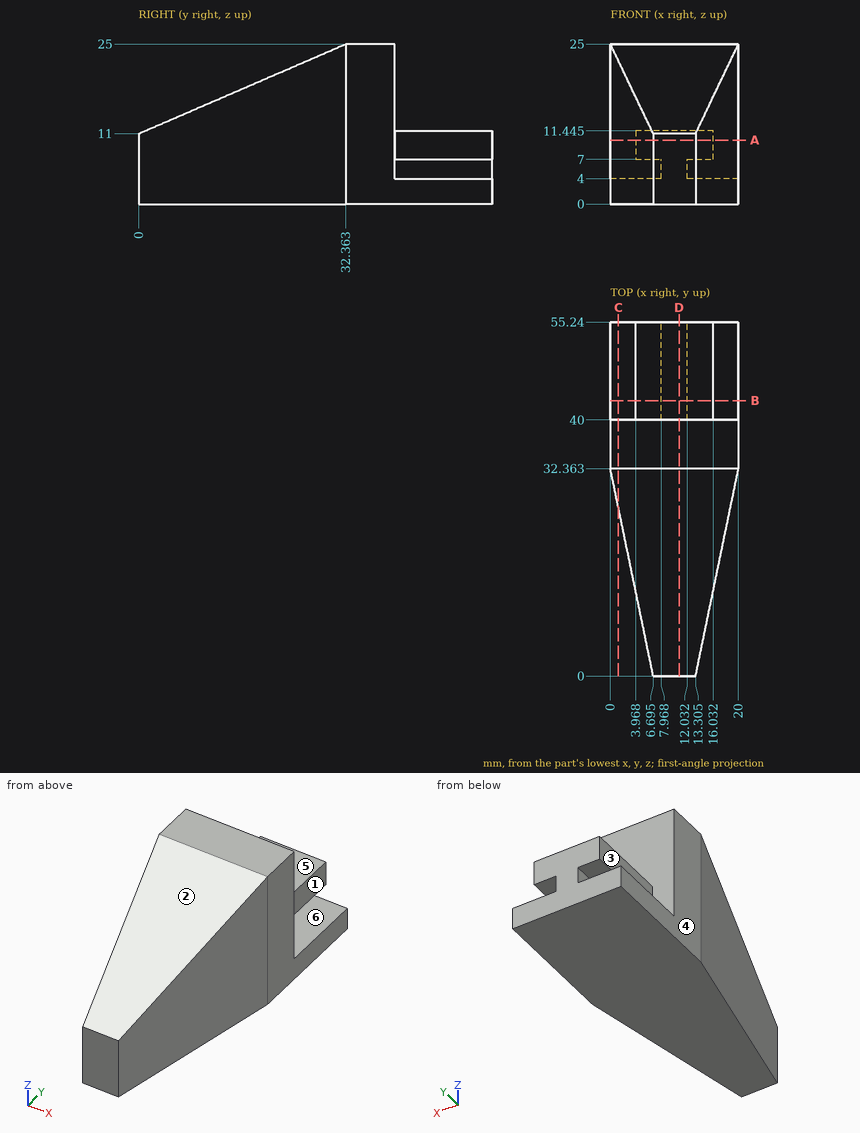
The figure shows three views and two pictorial views of one solid part (mm, origin at its lowest corner). Answer the questions. A direction names the side the tool comes from. Round coordinates to 2 decimals unless told otherwise and drop trailing zeros. Order: outer loops, then holes, each group sorted by start corner. A loop starts at its lowest first (then second) coordinate and runs counter-clockwise, first axis right, second up. Notation, with made-up numbers: M 8,-2 L 27,-2 A36 cw 27,35 Z; hole C 55,50 d4. An arc over 180 degrees is marked long. Answer in a Markdown table with one row per item. Add a question column.
1) Which of the six approach directions +Z, -Z, +X, -X, +Y, -Y give full straight-line access (tool end or side, diameter ignored) to the marked faces 1, 2 and 3?
2) Flat-ended cylindrical pins translate along their axes: pin 1 Ø8 at (x, z) = (2.5, 22.5) entering from +Y; pin 2 Ø4.5 at (x, y) = (6.5, 44.5) entering from -Z; pin 3 Ø6.5 at (x, y) = (15, 44) entering from +Z (1 decimal); pin 4 Ø0.9 at (y, z) = (46.5, 6) entering from -X. Find the tip coordinate at first contact, or state that the pin passes through.
3) The part is cut by section B-B on y = 43. Determine the outline of the cut face in (x, z) (1 decimal).
4) The part is cut by section C-C on x = 1.25. Determine the outline of the cut face in (y, z), plus the area to 3 significant figures.
5) The part is cut by section A-A on z = 10. Determine the outline of the cut face in (x, y) (1 decimal).
6) The part is cut by section D-D on x = 10.75. Determine the outline of the cut face in (y, z) (1 decimal), plus the area to 3 significant figures.
7) Consider line 1 along Z through (x, y) = (6, 52.5) (1 decimal); line 2 along X through (y, z) = (41.5, 10.25); line 3 along Z through (x, y) = (16, 14.5). Determine where each line is inside the solid, lowest interval first. Write a range as from..to.
8) Determine the mould class of the marked faces 4, 5 and 6 for opening direction Z: pulls with the +Z half, pulls with the -Z half, needs draft (parallel to the pull), parting line crosses it, or undercut.
Findings below:
| question | item | result |
|---|---|---|
| 1 | face 1 | +Z, +X, +Y |
| 1 | face 2 | +Z, +X, -X, -Y |
| 1 | face 3 | +Z, -X, +Y |
| 2 | pin 1 | stops at y = 40 |
| 2 | pin 2 | stops at z = 0 |
| 2 | pin 3 | stops at z = 11.4 |
| 2 | pin 4 | stops at x = 7.97 |
| 3 | outline | M 0,0 L 20,0 L 20,4 L 12,4 L 12,7 L 16,7 L 16,11.4 L 4,11.4 L 4,7 L 8,7 L 8,4 L 0,4 Z |
| 4 | outline | M 26.32,0 L 55.24,0 L 55.24,4 L 40,4 L 40,25 L 32.36,25 L 26.32,22.39 Z |
| 4 | area | 395 mm² |
| 5 | outline | M 0,32.4 L 6.7,0 L 13.3,0 L 20,32.4 L 20,40 L 16,40 L 16,55.2 L 4,55.2 L 4,40 L 0,40 Z |
| 6 | outline | M 0,0 L 55.2,0 L 55.2,11.4 L 40,11.4 L 40,25 L 32.4,25 L 0,11 Z |
| 6 | area | 948 mm² |
| 7 | line 1 | z = 0..4, 7..11.4 |
| 7 | line 2 | x = 3.97..16.03 |
| 7 | line 3 | z = 0..17.27 |
| 8 | face 4 | needs draft |
| 8 | face 5 | pulls with the +Z half |
| 8 | face 6 | undercut |
